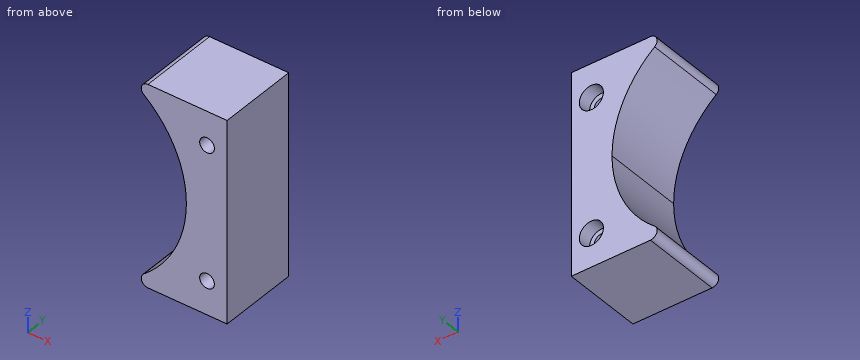
```python
from build123d import *

# Parameters (mm, degrees)
F0_W           = 75
F0_H           = 150
F1_DEPTH       = 30
F3_DEPTH       = 60.001
F5_D           = 11
F5_CBORE_D     = 18
F5_CBORE_DEPTH = 10


with BuildPart() as f1:
    # F0 (on Front) → F1 (new body, symmetric)
    with BuildSketch(Plane.XZ):
        Rectangle(F0_W, F0_H)
    extrude(amount=F1_DEPTH, both=True)

    # F2 (on face) → F3 (cut, through all)
    with BuildSketch(Plane.XZ.offset(30)):
        with BuildLine():
            ThreePointArc((-24.768539, -66.091569), (-1.31881, -36.675997), (7.05, 0))
            ThreePointArc((7.05, 0), (-1.31881, 36.675997), (-24.768539, 66.091569))
            ThreePointArc((-24.768539, 66.091569), (-162.05, 0), (-24.768539, -66.091569))
        make_face()
        with BuildLine():
            ThreePointArc((-37.5, 74.489613), (-30.944519, 70.578253), (-24.768539, 66.091569))
            ThreePointArc((-24.768539, 66.091569), (-26.369403, 71.651945), (-21.650179, 75))
            Line((-21.650179, 75), (-37.5, 75))
            Line((-37.5, 75), (-37.5, 74.489613))
        make_face()
        with BuildLine():
            ThreePointArc((-21.650179, -75), (-26.369403, -71.651945), (-24.768539, -66.091569))
            ThreePointArc((-24.768539, -66.091569), (-30.944519, -70.578253), (-37.5, -74.489613))
            Line((-37.5, -74.489613), (-37.5, -75))
            Line((-37.5, -75), (-21.650179, -75))
        make_face()
    extrude(amount=-F3_DEPTH, mode=Mode.SUBTRACT)

    # F5 (through all)
    with Locations(Plane(origin=(0, 30, 0), x_dir=(-1, 0, 0), z_dir=(0, 1, 0))):
        with Locations((-22.5, 50), (-22.5, -50)):
            CounterBoreHole(F5_D / 2, F5_CBORE_D / 2, F5_CBORE_DEPTH)


solid = f1.part
```
Can you work these out from the model? Positions are in its coordinate system, mm. Give positions to 0.01 mm unless a question says otherwise; leave off trailing zeros. Order: outer loops, then holes, each group sorted by start corner. A loop starts at its lowest first (then second) coordinate and runs counter-clockwise, first axis right, second up. Notation, with made-up numbers: M 20.25,-37 L 53.25,-37 A34 cw 53.25,-5 Z; hole C 17,-29 d2. An arc over 180 degrees is marked long. Write item = value, one per line. Start each with the question number.
Q1. Suppose I cut it at B-B (x = -9.5). Write out the boundary of the cut face in (y, z).
Q2. Will these pins go through, and if not, where does the flat tip stop? pin 1 Ø9 at (x, z) = (22, -48) entering from +Y; pin 2 Ø6.5 at (x, z) = (22.5, 50) entering from -Y.
Q3. Suppose I cut it at C-C (y = 5.5). Write out the boundary of the cut face in (x, z).
Q4. Suppose I cut it at D-D (z = 50). Write out the boundary of the cut face in (x, y).
Q5. I need wall thicknesses on probe 1 along Z at (x, y) = (22.5, 28); probe 2 along Z at (x, y) = (14.5, 27); probe 3 along Z at (x, y) = (-7.5, 22.5). Which ranges of each line are inside material? Lowest first, please. Write a range as [from, to].
Q6. Suppose I cut it at A-A (x = 22.5). Write out the boundary of the cut face in (y, z), plus the area to 3 significant figures.
Check result:
q1.outline = M -30,-75 L 30,-75 L 30,-50.25 L -30,-50.25 Z; M -30,50.25 L 30,50.25 L 30,75 L -30,75 Z
q2.pin_1 = 20
q2.pin_2 = through
q3.outline = M -24.77,-66.09 A5 ccw -21.65,-75 L 37.5,-75 L 37.5,75 L -21.65,75 A5 ccw -24.77,66.09 A84.55 cw 7.05,0 A84.55 cw Z; hole C 22.5,-50 d11; hole C 22.5,50 d11
q4.outline = M -9.32,-30 L 17,-30 L 17,20 L 13.5,20 L 13.5,30 L -9.32,30 Z; M 28,-30 L 37.5,-30 L 37.5,30 L 31.5,30 L 31.5,20 L 28,20 Z
q5.probe_1 = [-75, -59], [-41, 41], [59, 75]
q5.probe_2 = [-75, -54.12], [-45.88, 45.88], [54.12, 75]
q5.probe_3 = [-75, -47.42], [47.42, 75]
q6.outline = M -30,-75 L 30,-75 L 30,-59 L 20,-59 L 20,-55.5 L -30,-55.5 Z; M -30,-44.5 L 20,-44.5 L 20,-41 L 30,-41 L 30,41 L 20,41 L 20,44.5 L -30,44.5 Z; M -30,55.5 L 20,55.5 L 20,59 L 30,59 L 30,75 L -30,75 Z
q6.area = 7,540 mm2
